from build123d import *

# Parameters (mm, degrees)
SM_BASE_FLANGE_1_DEPTH = 20
CHAMFER_1_SIZE         = 3
SKETCH_6_R             = 1.6
CUT_EXTRUDE_1_DEPTH    = 52.23475383
PATTERN_LINEAR_1_COUNT = 2
PATTERN_LINEAR_1_PITCH = 10
SKETCH_7_R             = 1.6
CUT_EXTRUDE_2_DEPTH    = 52.23475383
PATTERN_LINEAR_2_COUNT = 2
PATTERN_LINEAR_2_PITCH = 8


# Sheet-metal steps are written as plain solids
with BuildPart() as part:
    # Sketch 1 → 基材-凸緣1 (new body)
    with BuildSketch(Plane.XY):
        with BuildLine():
            Line((0, 40), (0, 3.7366))
            ThreePointArc((0, 3.7366), (1.094424801, 1.094424801), (3.7366, 0))
            Line((3.7366, 0), (25, 0))
            Line((25, 0), (25, 3))
            Line((25, 3), (3.7366, 3))
            ThreePointArc((3.7366, 3), (3.215745145, 3.215745145), (3, 3.7366))
            Line((3, 3.7366), (3, 40))
            Line((3, 40), (0, 40))
        make_face()
    extrude(amount=SM_BASE_FLANGE_1_DEPTH)

    # 導角1
    chamfer_1_edges = [part.edges().sort_by_distance(p)[0] for p in [
        (25, 1.5, 20),
        (25, 1.5, 0),
        (1.5, 40, 20),
        (1.5, 40, 0),
    ]]
    chamfer(chamfer_1_edges, length=CHAMFER_1_SIZE)

    # 草圖6 → 除料-伸長1 (cut, through all)
    with BuildSketch(Plane.XZ):
        with Locations(Location((20, 10, 0), (0, 0, 270))):
            Circle(SKETCH_6_R)
    cut_extrude_1 = extrude(amount=-CUT_EXTRUDE_1_DEPTH, mode=Mode.SUBTRACT)

    # 直線複製排列1: 除料-伸長1 ×2
    with Locations(*[(-i * PATTERN_LINEAR_1_PITCH, 0, 0) for i in range(1, PATTERN_LINEAR_1_COUNT)]):
        add(cut_extrude_1, mode=Mode.SUBTRACT)

    # 草圖7 → 除料-伸長2 (cut, through all)
    with BuildSketch(Plane.ZY):
        with Locations((10, 36)):
            Circle(SKETCH_7_R)
    cut_extrude_2 = extrude(amount=-CUT_EXTRUDE_2_DEPTH, mode=Mode.SUBTRACT)

    # 直線複製排列2: 除料-伸長2 ×2
    with Locations(*[(0, -i * PATTERN_LINEAR_2_PITCH, 0) for i in range(1, PATTERN_LINEAR_2_COUNT)]):
        add(cut_extrude_2, mode=Mode.SUBTRACT)


solid = part.part
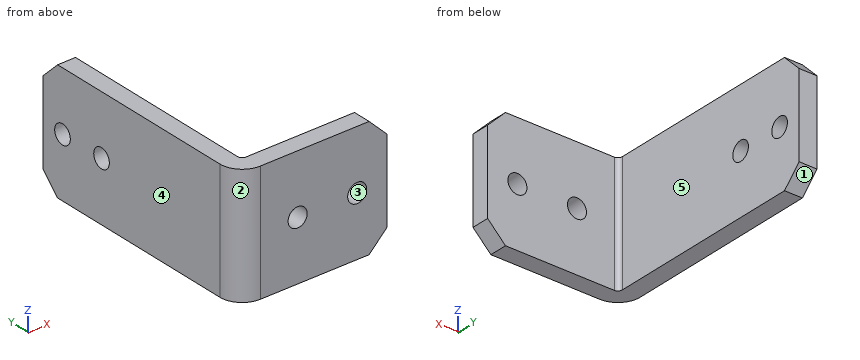
Source: CAD feature listing. Evaluate the final solid. Frame: model axes, mm. Face numbers are marked on the shaded views. A direction names the side the tool comes from. Round coordinates to 2 decimals unless told otherwise and drop trailing zeros. Loops run counter-clockwise (first coordinate to the right, second up) from the corner with the lowest first, then second, coordinate; pieces in that order, holes last. Notation, with made-up numbers: (80.25, 1.5) -> (89.25, 1.5) arc R28 ccw to (89.25, 31.5) -> close; hole circle Ø2 at (47.5, 56.25). An arc over 180 degrees is marked (long way). Answer as a JSON object with one key per item and string values. Group by question number.
Q1. Section query B-B (x = 20). Output: boundary loops of the cut face in (y, z).
Q2. Section query A-A (z = 10). Output: boundary loops of the cut face in (x, y).
Q3. Mould query, pull axis Z, two halves, no side actions, for the marked faces 1, 2 and 3. Classes: pulls with the +Z half, pulls with the -Z half, needs draft (parallel to the pull), parting line crosses it, or undercut.
Q4. Access query for the marked faces 4 and 5. Directions: +Z, -Z, +X, -X, +Y, -Y. A direction counts if a zero-diameter tool reaches every point of the face in a straight line with its end or side. Return the directions, or none.
Q5. Ray query, line 1 (X direction, y = 2.4, z = 10); line 2 (X direction, y = 1.3, z = 10); line 3 (Y direction, x = 1.25, z = 10). Return the intervals inside material, ascending. Write a range as from..to.
Q6. Section query D-D (z = 5.75). Output: boundary loops of the cut face in (x, y).
Q7. Contact query for flat-ended pins moving along their axis: P1, Ø2.5, axis at y = 28, z = 10, coming from the -X side; P2, Ø3, axis at x = 6.5, z = 5.5, coming from the +Y side; P3, Ø3, axis at y = 5, z = 7, coming from the +X side. Output: stop coordinate, or through.
Completed:
{
 "1": {"outline": "(0, 0) -> (3, 0) -> (3, 8.4) -> (0, 8.4) -> close; (0, 11.6) -> (3, 11.6) -> (3, 20) -> (0, 20) -> close"},
 "2": {"outline": "(0, 3.74) arc R3.74 ccw to (3.74, 0) -> (8.4, 0) -> (8.4, 3) -> (3.74, 3) arc R0.74 cw to (3, 3.74) -> (3, 26.4) -> (0, 26.4) -> close; (0, 29.6) -> (3, 29.6) -> (3, 34.4) -> (0, 34.4) -> close; (0, 37.6) -> (3, 37.6) -> (3, 40) -> (0, 40) -> close; (11.6, 0) -> (18.4, 0) -> (18.4, 3) -> (11.6, 3) -> close; (21.6, 0) -> (25, 0) -> (25, 3) -> (21.6, 3) -> close"},
 "3": {"face 1": "pulls with the -Z half", "face 2": "needs draft", "face 3": "undercut"},
 "4": {"face 4": "+Z, -Z, -X, +Y, -Y", "face 5": "+Z, -Z, +X, +Y"},
 "5": {"line 1": "0.25..8.4, 11.6..18.4, 21.6..25", "line 2": "0.9..8.4, 11.6..18.4, 21.6..25", "line 3": "0.95..26.4, 29.6..34.4, 37.6..40"},
 "6": {"outline": "(0, 3.74) arc R3.74 ccw to (3.74, 0) -> (25, 0) -> (25, 3) -> (3.74, 3) arc R0.74 cw to (3, 3.74) -> (3, 40) -> (0, 40) -> close"},
 "7": {"P1": "through", "P2": "y = 3", "P3": "x = 3.04"}
}
